Build history of the part. All positions in model axes, mm. Face numbers are marked on the shaded views. A direction names the side the tool comes from. Give positions to 0.01 mm unless a question says otherwise; leave off trailing zeros. Write each loop counter-clockwise with the first axis right and the second up, starting at its lowest first coordinate (ties: lowest second). Pieces come first, ordered by that corner, then holes. Notation, with made-up numbers: (-1.5, 36.25) - (50.5, 36.25) arc R28 ccw to (50.5, 75.25) - close; hole circle Ø3 at (25.5, -3.75). An arc over 180 degrees is marked (long way). Use one line per item in the form item = value. Start each with the question number.
from build123d import *

# Parameters (mm, degrees)
F0_R     = 2.5
F1_DEPTH = 10
F0_R_2   = 4.5
F2_DEPTH = 3
F3_R     = 2.6
F5_DEPTH = 2


with BuildPart() as f1:
    # F0 (on Top) → F1 (new body)
    with BuildSketch(Plane.XY):
        Circle(F0_R)
    extrude(amount=-F1_DEPTH)

    # F0 (on Top) → F2 (join)
    with BuildSketch(Plane.XY):
        Circle(F0_R_2)
        Circle(F0_R, mode=Mode.SUBTRACT)
        Circle(F0_R)
    extrude(amount=F2_DEPTH)

    # F3
    f3_edges = [f1.edges().sort_by_distance(p)[0] for p in [
        (-4.5, 0, 3),
    ]]
    fillet(f3_edges, radius=F3_R)

    # F4 (on face) → F5 (cut)
    with BuildSketch(Plane.XY.offset(3)):
        Polygon((-0.866025, -1.5), (0.866025, -1.5), (1.732051, 0), (0.866025, 1.5), (-0.866025, 1.5), (-1.732051, 0), align=None)
    extrude(amount=-F5_DEPTH, mode=Mode.SUBTRACT)


solid = f1.part
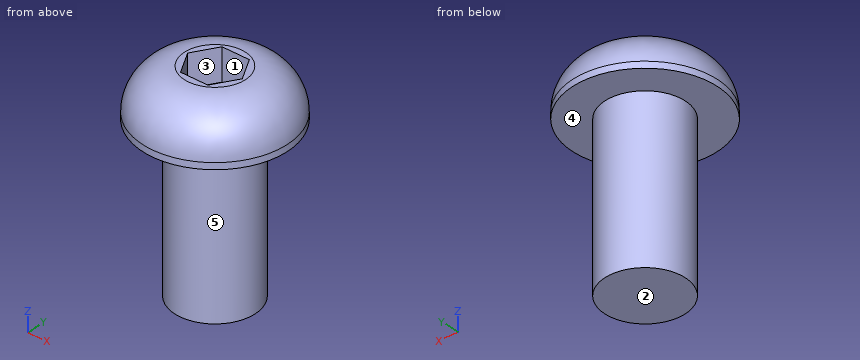
(1) Two-plate mould, pull along Y, no slides. Class the marked faces 3, 4 and 5: +Y half, -Y half, draft (parallel to the pull), parting line (faces both ways), or undercut.
(2) Which spindle directions (+Z, -Z, +X, -X, +Y, -Y) get a long thin tool onto all of the face, cutting with end or side? Do the marked faces 1 and 2. Say none if no direction does.
(3) Cut at A-A, the plane z = -5.5. Give the cut face in (x, y).
(4) Wall check: line 1 (Z direction, x = -1.75, y = 1); line 2 (Y direction, x = 0.75, z = 2.5); line 3 (Z direction, x = 0.25, y = 0.75). Give the ranges that are in metal, low to high. Write a range as from..to.
(5) Pin check, flat tips, straight feed: pin 1 Ø1.4 at (x, z) = (-0.5, 2.5) entering from +Y; pin 2 Ø0.9 at (x, z) = (0, 2) entering from -Y; pin 3 Ø0.9 at (x, y) = (0.5, 0.5) entering from +Z; pin 4 Ø3 at (x, y) = (-1, -2.5) entering from +Z. Stop position of each tip, or through.
Solution:
q1.face_3 = undercut
q1.face_4 = draft
q1.face_5 = parting line
q2.face_1 = +Z
q2.face_2 = -Z, +X, -X, +Y, -Y
q3.outline = circle Ø5 at (0, 0)
q4.line_1 = -10..3
q4.line_2 = -3.35..-1.5, 1.5..3.35
q4.line_3 = -10..1
q5.pin_1 = 4.07
q5.pin_2 = -4.23
q5.pin_3 = 1
q5.pin_4 = 3
